Autodesk Inventor part; units mm, degrees
ref_plane "Work Plane1" through (46, 0, 0) normal (1, 0, 0) x (0, 1, 0)
ref_plane "XZ Plane" through (0, 0, 0) normal (0, 1, 0) x (-1, 0, 0)
ref_plane "XY Plane" through (0, 0, 0) normal (0, 0, 1) x (1, 0, 0)
sketch "Sketch1" plane through (0, 0, 0) normal (0, 1, 0) x (-1, 0, 0)
  circle A0 centre (0, 0) radius 46
  circle A1 centre (0, 0) radius 38.445
  circle A2 centre (0, 0) radius 11.5
  dimension "d0" = 92
  dimension "d1" = 76.89
  dimension "d2" = 23
extrude "Extrusion1" add sketch "Sketch1" against normal blind 65 contours A1
extrude "Extrusion2" add sketch "Sketch1" along normal blind 50 contours A0 | A1
sketch "Sketch2" plane through (0, 0, 0) normal (1, 0, 0) x (0, 1, 0)
  line L0 (50, -46) -> (50, 46)
  line L1 (0, -46) -> (0, 46)
  line L2 (-65, 38.445) -> (-65, -38.445)
  line L3 (0, -38.445) -> (0, 38.445)
  line L4 (0, -46) -> (0, -38.445)
  line L5 (0, -38.445) -> (-65, -38.445)
  line L6 (-65, -38.445) -> (-65, -11.5)
  line L7 (-65, -11.5) -> (50, -11.5)
  line L8 (50, -11.5) -> (50, -46)
  line L9 (0, 38.445) -> (0, 46)
  line L10 (50, 46) -> (50, 11.5)
  line L11 (50, 11.5) -> (-65, 11.5)
  line L12 (-65, 11.5) -> (-65, 38.445)
  line L13 (-65, 38.445) -> (0, 38.445)
  line L14 (45, 46) -> (40, 46)
  line L15 (40, 46) -> (40, 43)
  line L16 (40, 43) -> (45, 43)
  line L17 (45, 43) -> (45, 46)
  line L18 (35, 46) -> (30, 46)
  line L19 (30, 46) -> (30, 43)
  line L20 (30, 43) -> (35, 43)
  line L21 (35, 43) -> (35, 46)
  line L22 (-65, 11.5) -> (50, 11.5)
  line L23 (6, -11.5) -> (6, 11.5)
  line L24 (6, 11.5) -> (-65, 30.5244)
  line L25 (-88, 0) -> (73, 0)
  line L26 (-65, 30.5244) -> (-65, 0)
  line L27 (-65, 0) -> (6, 0)
  line L28 (7, 11.5) -> (7, -11.5)
  line L29 (7, 11.5) -> (50, 36.3261)
  line L30 (50, 36.3261) -> (50, 0)
  line L31 (7, 0) -> (50, 0)
  line L32 (50, -46) -> (0, -46)
  line L33 (0, 46) -> (50, 46)
  point P0 (0, 0)
  point P1 (30, 46)
  point P2 (0, 13.1077)
  point P3 (0, 0)
  dimension "d11" = 5
  dimension "d12" = 5
  dimension "d13" = 5
  dimension "d14" = 5
  dimension "d15" = 3
  dimension "d16" = 71
  dimension "d17" = 15
  dimension "d18" = 1
  dimension "d19" = 30
revolve "Revolution1" cut sketch "Sketch2" angle 360 about axis through (0, -10, 0) along (0, 1, 0) contours L25 L28 L11 L0 | L11 L29 L0 | L25 L1 L11 L23 | L25 L2 L11 L1 | L11 L1 L24 | L11 L2 L24 L1 | L17 L16 L15 L14 | L21 L20 L19 L18
ref_plane "Work Plane1" through (46, 0, 0) normal (1, 0, 0) x (0, 1, 0)
sketch "Sketch3" plane through (46, 0, 0) normal (1, 0, 0) x (0, 1, 0)
  line L0 (45, 0) -> (50, 0)
  line L1 (35, 0) -> (40, 0)
  line L2 (0, 0) -> (30, 0)
  circle A0 centre (15, 0) radius 3.5
  line L3 (0, -46) -> (0, 46)
  dimension "d23" = 7
  dimension "d24" = 15
extrude "Extrusion3" cut sketch "Sketch3" against normal blind 23
pattern_circular "Circular Pattern1" count 8 over 360 about axis through (0, 0, 0) along (0, 1, 0) of "Extrusion3"
properties part number "nozzle 94mm"
Can you work these out from the model? Positions are in its coordinate system, mm. A direction names the side the tool comes from. Coordinates: 2 decimals unless noted, no trailing zeros. Write each loop counter-clockwise with the first axis right and the second up, starting at its lowest first coordinate (ties: lowest second). Pieces come first, ordered by that corner, then holes. Notation, with made-up numbers: (34.25, 48) -> (38.25, 48) arc R15 ccw to (38.25, 70) -> close; hole circle Ø10 at (70.25, 18). An arc over 180 degrees is marked (long way). Write each question's results on one line, items separated by ' | '. Start each with the question number.
Q1. If I drill on probe 1 along Y at (x, z) = (38, 0); probe 2 along Z at (x, y) = (-28.5, 15); probe 3 along X at (y, z) = (6, 0), over which ranges is the centre line in solid material (lowest first)?
Q2. Imagine slicing it at B-B (z = 27.5). State how many separate pieces and enclosed holes the cut face has, then the cut area to 3 significant figures.
Q3. Imagine slicing it at C-C (y = -35). Write out the boundary of the cut face in (x, z) (3 decimals), then the cut area to 3 significant figures.
Q4. I'm going to push flat-ended pins straight in: pin 1 (6 mm diameter, centred on y = 16, z = -6, fed in from -X); pin 2 (4 mm diameter, centred on x = 3, y = -46, fed in from +Z); pin 3 (6.5 mm diameter, centred on y = 15, z = 0, fed in from -X); pin 4 (18.5 mm diameter, centred on x = 0, z = 0, fed in from -Y). Where does each tip first touch, or does it pass through?
Q5. On a 3-axis mill with a long thin cutter (end or side, diameter ignored), from which of +Z, -Z, +X, -X, +Y, -Y can I reach the whole of each face in a straight line? I mean faces 4 (the face through (-1.05, 18.34, 34.66)), 5 (the face through (-36.67, -32.04, 11.55)), 6 (the face through (-27, 35, 34)), 7 (the face through (34.66, 18.34, 1.05)). Say none if no direction works.
Q6. We'd pull the mould along X, two halves only. Please class faces 1 (the face through (-34, 50, 14)), 2 (the face through (42.634, 42.535, -5.598)), 3 (the face through (1.5, 6.5, -11.4)): +X half, -X half, draft (parallel to the pull), parting line (faces both ways), or undercut.
Taken from the geometry:
1) probe 1: y = -65 to 11.5, 18.5 to 50 | probe 2: z = -36.11 to -33.45, -23.55 to -3.5, 3.5 to 23.55, 33.45 to 36.11 | probe 3: x = -46 to -11.5, 11.5 to 46
2) separate pieces: 1 | enclosed holes: 3 | area: 6,290 mm^2
3) outline: circle Ø76.89 at (0, 0); hole circle Ø44.972 at (0, 0) | area: 3,050 mm^2
4) pin 1: stops at x = -45.9 | pin 2: stops at z = 38.43 | pin 3: stops at x = -23 | pin 4: passes through
5) face 4: +Z | face 5: -Y | face 6: none | face 7: +X
6) face 1: draft | face 2: parting line | face 3: undercut
